The drawing under review shows one solid part. Ordinate dimensions are in mm from its lowest x, y, z. A direction names the side the tool comes from. Coordinates: 2 decimals unless noted, no trailing zeros. Order: outer loops, then holes, each group sorted by start corner. A loop starts at its lowest first (then second) coordinate and runs counter-clockwise, first axis right, second up. Notation, with made-up numbers: (-23, 43) - (10, 43) arc R27 ccw to (10, 72) - close; hole circle Ø8 at (67.25, -4). An arc over 180 degrees is marked (long way). Answer in a Markdown table with one row per item.
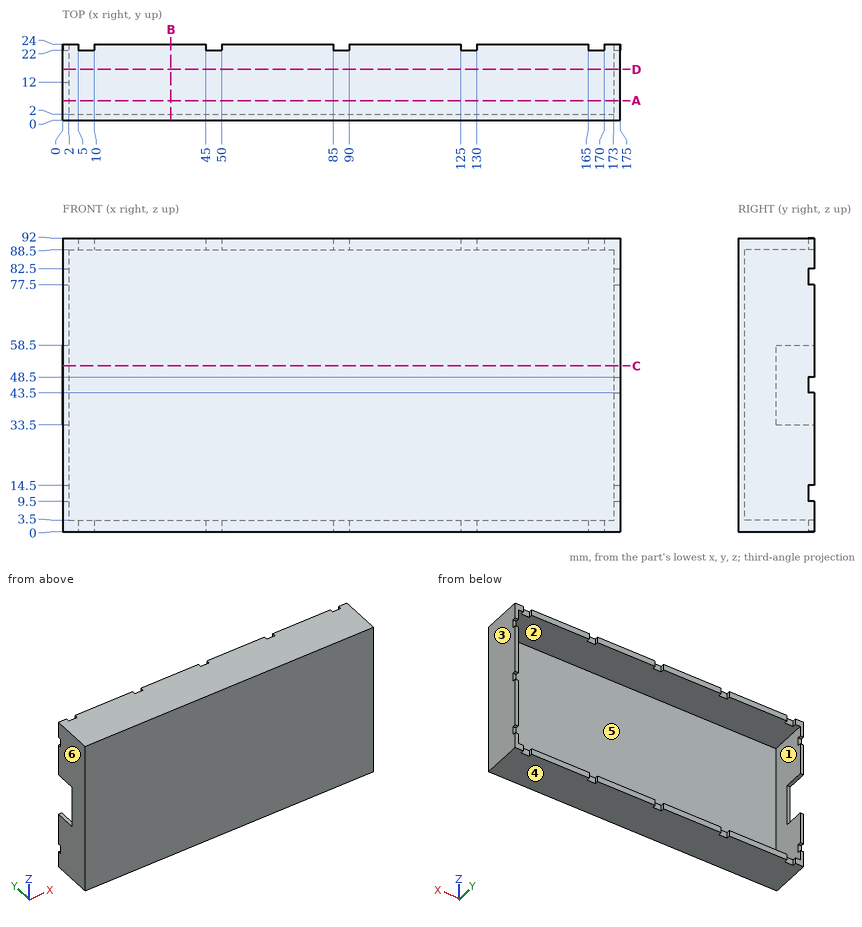
Item 1: We need section C-C, the plane z = 52. Write out the cut boundary in (x, y), then the cut area to 3 significant figures.
Check values:
| item | result |
|---|---|
| outline | (0, 0) - (175, 0) - (175, 24) - (173, 24) - (173, 2) - (2, 2) - (2, 12) - (0, 12) - close |
| area | 414 mm^2 |
Item 2: We need section A-A, the plane y = 6.25. Write out the cut boundary in (x, z), then the cut area to 4 significant figures.
Check values:
| item | result |
|---|---|
| outline | (0, 0) - (175, 0) - (175, 92) - (0, 92) - close; hole (2, 3.5) - (173, 3.5) - (173, 88.5) - (2, 88.5) - close |
| area | 1,565 mm^2 |
Item 3: We need section B-B, the plane x = 34. Write out the cut boundary in (y, z), then the cut area to 3 significant figures.
Check values:
| item | result |
|---|---|
| outline | (0, 0) - (24, 0) - (24, 3.5) - (2, 3.5) - (2, 88.5) - (24, 88.5) - (24, 92) - (0, 92) - close |
| area | 338 mm^2 |
Item 4: We need section D-D, the plane y = 16. Write out the cut boundary in (x, z), then the cut area to 4 significant figures.
Check values:
| item | result |
|---|---|
| outline | (0, 0) - (175, 0) - (175, 92) - (0, 92) - (0, 58.5) - (2, 58.5) - (2, 88.5) - (173, 88.5) - (173, 3.5) - (2, 3.5) - (2, 33.5) - (0, 33.5) - close |
| area | 1,515 mm^2 |
Item 5: Tool access review of the marked faces 5 and 6: name each direction out of +Z, -Z, +X, -X, +Y, -Y from which nothing blocks a thin tool from reaching the whole face with its end or side.
Check values:
| item | result |
|---|---|
| face 5 | +Y |
| face 6 | +Z, -Z, -X, +Y, -Y |
Item 6: To check wall thickness, follow line 1 (Z direction, x = 10, y = 3.5); line 2 (X direction, y = 2.25, z = 13); line 3 (X direction, y = 19.75, z = 48.5). State the ranges of each line that lie inside material, in increasing order. Write a range as from..to.
Check values:
| item | result |
|---|---|
| line 1 | 0..3.5, 88.5..92 |
| line 2 | 0..2, 173..175 |
| line 3 | 173..175 |
Item 7: Clearance check with flat-ended pins moving along their axes: pin 1 Ø3 at (y, z) = (18.5, 16.5) entering from -X; pin 2 Ø1 at (x, z) = (48, 1.5) entering from +Y; pin 3 Ø2 at (x, z) = (53, 12.5) entering from +Y. State where each tip first meets the part, or that it passes through.
Check values:
| item | result |
|---|---|
| pin 1 | x = 0 |
| pin 2 | y = 22 |
| pin 3 | y = 2 |
Item 8: Mouldability with a two-part tool opening along Z and no side actions: class the marked faces 1, 2, 3 and 4 as +Z half, -Z half, draft (parallel to the pull), parting line (faces both ways), or undercut.
Check values:
| item | result |
|---|---|
| face 1 | undercut |
| face 2 | undercut |
| face 3 | draft |
| face 4 | -Z half |
